Model file for the job. Use its own axes, mm. A direction names the side the tool comes from. Round coordinates to 2 decimals unless told otherwise and drop trailing zeros. Loops run counter-clockwise (first coordinate to the right, second up) from the corner with the lowest first, then second, coordinate; pieces in that order, holes last. Notation, with made-up numbers: (27, 44) - (69, 44) arc R24 ccw to (69, 69) - close; hole circle Ø8 at (29.25, -19.75). An arc over 180 degrees is marked (long way). Use one line per item in the form item = value.
from build123d import *

# Parameters (mm, degrees)
F0_W     = 13
F0_H     = 13
F1_DEPTH = 20
F2_W     = 13
F2_H     = 13
F3_DEPTH = 15
F5_DEPTH = 7
F7_DEPTH = 8
F9_DEPTH = 17


with BuildPart() as f1:
    # F0 (on Top) → F1 (new body)
    with BuildSketch(Plane.XY):
        with Locations((6.5, 6.5)):
            Rectangle(F0_W, F0_H)
    extrude(amount=F1_DEPTH)

    # F2 (on face) → F3 (join)
    with BuildSketch(Plane.XY.offset(20)):
        Polygon((-2, 15), (-2, 0), (-2, -2), (15, -2), (15, 15), align=None)
        with Locations((6.5, 6.5)):
            Rectangle(F2_W, F2_H, mode=Mode.SUBTRACT)
    extrude(amount=-F3_DEPTH)

    # F4 (on face) → F5 (cut)
    with BuildSketch(Plane.YZ.offset(15)):
        with BuildLine():
            ThreePointArc((7.5, 13), (7.207107, 13.707107), (6.5, 14))
            ThreePointArc((6.5, 14), (5.792893, 12.292893), (7.5, 13))
        make_face()
    extrude(amount=-F5_DEPTH, mode=Mode.SUBTRACT)

    # F6 (on face) → F7 (cut)
    with BuildSketch(Plane(origin=(-2, 0, 0), x_dir=(0, -1, 0), z_dir=(-1, 0, 0))):
        with BuildLine():
            ThreePointArc((-4, 16), (-4.732233, 17.767767), (-6.5, 18.5))
            ThreePointArc((-6.5, 18.5), (-8.267767, 14.232233), (-4, 16))
        make_face()
    extrude(amount=-F7_DEPTH, mode=Mode.SUBTRACT)

    # F8 (on face) → F9 (cut)
    with BuildSketch(Plane(origin=(0, 0, 0), x_dir=(1, 0, 0), z_dir=(0, 0, -1))):
        with BuildLine():
            ThreePointArc((7.5, -6.5), (4.5, -3.5), (1.5, -6.5))
            ThreePointArc((1.5, -6.5), (4.5, -9.5), (7.5, -6.5))
        make_face()
    extrude(amount=-F9_DEPTH, mode=Mode.SUBTRACT)


solid = f1.part
1. Wall check: probe 1 along Z at (x, y) = (11.25, 6.5); probe 2 along Z at (x, y) = (13.25, 6.5); probe 3 along Y at (x, z) = (12.5, 13). Give the ranges that are in metal, low to high.
Geometry check:
probe_1 = 0 to 12, 14 to 20
probe_2 = 5 to 12, 14 to 20
probe_3 = -2 to 5.5, 7.5 to 15
2. Cut at B-B, the plane x = 11. Give the cut face in (y, z), plus the area to 3 significant figures.
Geometry check:
outline = (-2, 5) - (0, 5) - (0, 0) - (13, 0) - (13, 5) - (15, 5) - (15, 20) - (-2, 20) - close; hole circle Ø2 at (6.5, 13)
area = 317 mm^2
3. Flat gauge pins, fed straight in: pin 1 (1.5 mm diameter, centred on x = 4, z = 3.5, fed in from -Y); pin 2 (3 mm diameter, centred on y = 6.5, z = 16, fed in from -X); pin 3 (1.5 mm diameter, centred on y = 6, z = 3, fed in from -X). Where does each tip first touch, or does it go through?
Geometry check:
pin_1 = 0
pin_2 = 6
pin_3 = 0
4. Cut at A-A, the plane z = 7.75. Give the cut face in (x, y), plus the area to 3 significant figures.
Geometry check:
outline = (-2, -2) - (15, -2) - (15, 15) - (-2, 15) - close; hole circle Ø6 at (4.5, 6.5)
area = 261 mm^2
5. Cut at C-C, the plane x = 4.5. Give the cut face in (y, z).
Geometry check:
outline = (-2, 5) - (0, 5) - (0, 0) - (3.5, 0) - (3.5, 17) - (4.21, 17) arc R2.5 cw to (8.79, 17) - (9.5, 17) - (9.5, 0) - (13, 0) - (13, 5) - (15, 5) - (15, 20) - (-2, 20) - close
6. Cut at D-D, the plane y = 0.5. Give the cut face in (x, z).
Geometry check:
outline = (-2, 5) - (0, 5) - (0, 0) - (13, 0) - (13, 5) - (15, 5) - (15, 20) - (-2, 20) - close
7. Pull direction Y, two halves, no side cores. Call faces 4 (the flat face through (-1, 7, 5)), 5 (the cylindrical face through (7.5, 6.6, 8.4)), 6 (the flat face through (6, 13, 2)): +Y half, -Y half, draft (parallel to the pull), parting line (faces both ways), or undercut.
Geometry check:
face_4 = draft
face_5 = undercut
face_6 = +Y half
8. Tool access for faces 1 (the flat face through (0, 6, 2)), 2 (the flat face through (8, 6, 13)), 3 (the flat face through (6.3, 6.5, 17)): list every direction of +Z, -Z, +X, -X, +Y, -Y with a clear straight run to the whole face (end or side of a thin tool).
Geometry check:
face_1 = -Z, -X, +Y, -Y
face_2 = +X
face_3 = -Z
